from build123d import *

# Parameters (mm, degrees)
CROQUIS3_R              = 20
SALIENTE_EXTRUIR1_DEPTH = 8
SALIENTE_EXTRUIR3_START = 8
CROQUIS4_R              = 4
SALIENTE_EXTRUIR3_DEPTH = 1.5
CROQUIS7_R              = 1.625
CORTAR_EXTRUIR2_DEPTH   = 30.393876913


with BuildPart() as part:
    # Croquis3 → Saliente-Extruir1 (new body)
    with BuildSketch(Plane(origin=(0, 0, 0), x_dir=(1, 0, 0), z_dir=(0, 1, 0))):
        with Locations(Location((0, 0, 0), (0, 0, 270))):
            Circle(CROQUIS3_R)
    extrude(amount=SALIENTE_EXTRUIR1_DEPTH)

    # Croquis4 → Saliente-Extruir3 (add)
    with BuildSketch(Plane(origin=(0, 0, 0), x_dir=(1, 0, 0), z_dir=(0, 1, 0)).offset(SALIENTE_EXTRUIR3_START)):
        with Locations(Location((0, 0, 0), (0, 0, 270))):
            Circle(CROQUIS4_R)
    extrude(amount=SALIENTE_EXTRUIR3_DEPTH)

    # Croquis7 → Cortar-Extruir2 (cut, through all)
    with BuildSketch(Plane(origin=(0, 8, 0), x_dir=(1, 0, 0), z_dir=(0, 1, 0))):
        with Locations(Location((-14, 0, 0), (0, 0, 270))):
            Circle(CROQUIS7_R)
        with Locations(Location((14, 0, 0), (0, 0, 270))):
            Circle(CROQUIS7_R)
        with Locations(Location((0, 14, 0), (0, 0, 270))):
            Circle(CROQUIS7_R)
        with Locations(Location((0, -14, 0), (0, 0, 270))):
            Circle(CROQUIS7_R)
    extrude(amount=-CORTAR_EXTRUIR2_DEPTH, mode=Mode.SUBTRACT)


solid = part.part
Work out the finished part from the listing and answer in its coordinate system (mm). A direction names the side the tool comes from. Round coordinates to 2 decimals unless told otherwise and drop trailing zeros. Order: outer loops, then holes, each group sorted by start corner. A loop starts at its lowest first (then second) coordinate and runs counter-clockwise, first axis right, second up. Notation, with made-up numbers: M -26.75,82.25 L 26.25,82.25 A21 ccw 26.25,92.25 Z; hole C 2.5,26 d2. An arc over 180 degrees is marked long. One line per item, written item: value.
Q1. Find section C-C on y = 0.5. Write down the section's boundary in (x, z) (3 decimals).
Derived:
outline: C 0,0 d40; hole C -14,0 d3.25; hole C 0,-14 d3.25; hole C 0,14 d3.25; hole C 14,0 d3.25
Q2. Determine the mould class of faces 3 (the face through (-19.524, 3.944, -4.336)), 4 (the face through (0.49, 4.06, -12.45)), 5 (the face through (0, 9.5, 0)), 6 (the face through (0.49, 4.06, 15.55)) for opening direction X: released by +X, released by -X, zero draft, split by the parting line, or undercut.
Derived:
face 3: split by the parting line
face 4: undercut
face 5: zero draft
face 6: undercut
Q3. Straight lines are drawn through the part: line 1 (X direction, y = 4, z = 0) (3 decimals); line 2 (Y direction, x = 7, z = 16); line 3 (X direction, y = 7, z = 14) (3 decimals). For each, find the intervals that lie inside material, in ascending order.
Derived:
line 1: -20 to -15.625, -12.375 to 12.375, 15.625 to 20
line 2: 0 to 8
line 3: -14.283 to -1.625, 1.625 to 14.283
Q4. Flat-ended cylindrical pins translate along their axes: pin 1 (1.5 mm diameter, centred on y = 4.5, z = -13, fed in from -X); pin 2 (3.5 mm diameter, centred on x = 0, z = -14, fed in from +Y); pin 3 (1.5 mm diameter, centred on y = 5.5, z = 1, fed in from -X). Find the tip coordinate at first contact, or state that the pin passes through.
Derived:
pin 1: x = -15.81
pin 2: y = 8
pin 3: x = -20
Q5. Find section D-D on x = 15. Write down the section's boundary in (y, z).
Derived:
outline: M 0,-13.23 L 8,-13.23 L 8,-1.28 L 0,-1.28 Z; M 0,1.28 L 8,1.28 L 8,13.23 L 0,13.23 Z
Q6. Find section B-B on x = 0. Write down the section's boundary in (y, z) (3 decimals).
Derived:
outline: M 0,-20 L 8,-20 L 8,-15.625 L 0,-15.625 Z; M 0,-12.375 L 8,-12.375 L 8,-4 L 9.5,-4 L 9.5,4 L 8,4 L 8,12.375 L 0,12.375 Z; M 0,15.625 L 8,15.625 L 8,20 L 0,20 Z
Q7. For faces 1 (the face through (-3.905, 8.74, -0.867)), 2 (the face through (0, 0, 0)), determine the directions among +Z, -Z, +X, -X, +Y, -Y from which every point of the face is accessible in a straight line to the end or side of a thin tool.
Derived:
face 1: +Y
face 2: +Z, -Z, +X, -X, -Y
Q8. Find section A-A on z = 0. Write down the section's boundary in (x, y) (3 decimals), then the cut area to 3 significant figures.
Derived:
outline: M -20,0 L -15.625,0 L -15.625,8 L -20,8 Z; M -12.375,0 L 12.375,0 L 12.375,8 L 4,8 L 4,9.5 L -4,9.5 L -4,8 L -12.375,8 Z; M 15.625,0 L 20,0 L 20,8 L 15.625,8 Z
area: 280 mm²
